from build123d import *

# Parameters (mm, degrees)
F0_W     = 50.8
F0_H     = 50.8
F1_DEPTH = 6.35
F2_W     = 50.8
F2_H     = 8.870684
F3_DEPTH = 6.604
F4_W     = 50.8
F4_H     = 50.8
F5_DEPTH = 6.35
F6_R     = 10.16
F6_R_2   = 8.255
F7_DEPTH = 50.8


with BuildPart() as f1:
    # F0 (on Top) → F1 (new body)
    with BuildSketch(Plane.XY):
        Rectangle(F0_W, F0_H)
    extrude(amount=F1_DEPTH)

    # F2 (on face) → F3 (join)
    with BuildSketch(Plane.XY.offset(6.35)):
        with Locations((0, 20.964658)):
            Rectangle(F2_W, F2_H)
    extrude(amount=F3_DEPTH)

    # F4 (on face) → F5 (join)
    with BuildSketch(Plane.XY.offset(12.954)):
        Rectangle(F4_W, F4_H)
    extrude(amount=F5_DEPTH)

    # F6 (on face) → F7 (join)
    with BuildSketch(Plane.XY.offset(19.304)):
        Circle(F6_R)
        Circle(F6_R_2, mode=Mode.SUBTRACT)
    extrude(amount=F7_DEPTH)


solid = f1.part
Geometry check sheet. Reference: the model listing, model coordinates, mm. A direction names the side the tool comes from. Round coordinates to 2 decimals unless told otherwise and drop trailing zeros. Order: outer loops, then holes, each group sorted by start corner. A loop starts at its lowest first (then second) coordinate and runs counter-clockwise, first axis right, second up. Notation, with made-up numbers: M 37,-33.75 L 51,-33.75 A21 cw 51,-23.75 Z; hole C 36,-30 d10. An arc over 180 degrees is marked long. Write each question's results on one line, items separated by ' | '. Start each with the question number.
1. Set-up check for faces 5 (the face through (0, -25.4, 3)), 6 (the face through (11, 0, 19.304)), 7 (the face through (0, -4, 6.35)): record each of +Z, -Z, +X, -X, +Y, -Y from which the full face is reachable in a straight line by a thin tool's end or side.
2. Cross-section at A-A on y = -19. Record the boundary of the cut face in (x, z), plus the area to 3 significant figures.
3. Cross-section at C-C on z = 32.5. Record the boundary of the cut face in (x, y) (3 decimals), plus the area to 3 significant figures.
4. Cross-section at B-B on x = 0. Record the boundary of the cut face in (y, z) (3 decimals), plus the area to 3 significant figures.
5. Go/stop test with flat-tipped pins: P1, Ø12, axis at y = 7.5, z = 58.5, coming from the +X side; P2, Ø3, axis at y = -10, z = 37.5, coming from the +X side; P3, Ø6, axis at x = -4.5, y = 18.5, coming from the +Z side. Record where each tip stops, or that it passes through.
6. Material ranges on L1, parallel to Y at x = 0, z = 49 (3 decimals); L2, parallel to Z at x = -5, y = 2; L3, parallel to X at y = -7, z = 42.5, recorded low to high. Write a range as from..to.
7. Cross-section at D-D on y = 0. Record the boundary of the cut face in (x, z) (3 decimals), plus the area to 3 significant figures.
8. Draft check along X on faces 1 (the face through (7.874, 2.48, 44.348)), 2 (the face through (0, 0, 19.304)), 3 (the face through (0, -25.4, 16)), 4 (the face through (25.4, 0, 14)). Enter one of: pulls with the +X half, pulls with the -X half, needs draft (parallel to the pull), parting line crosses it, or undercut.
Resolved:
1) face 5: +Z, -Z, +X, -X, -Y | face 6: +Z | face 7: +X, -X, -Y
2) outline: M -25.4,0 L 25.4,0 L 25.4,6.35 L -25.4,6.35 Z; M -25.4,12.95 L 25.4,12.95 L 25.4,19.3 L -25.4,19.3 Z | area: 645 mm2
3) outline: C 0,0 d20.32; hole C 0,0 d16.51 | area: 110 mm2
4) outline: M -25.4,0 L 25.4,0 L 25.4,19.304 L 10.16,19.304 L 10.16,70.104 L 8.255,70.104 L 8.255,19.304 L -8.255,19.304 L -8.255,70.104 L -10.16,70.104 L -10.16,19.304 L -25.4,19.304 L -25.4,12.954 L 16.529,12.954 L 16.529,6.35 L -25.4,6.35 Z | area: 897 mm2
5) P1: x = 10.05 | P2: x = 5.57 | P3: z = 19.3
6) L1: -10.16..-8.255, 8.255..10.16 | L2: 0..6.35, 12.95..19.3 | L3: -7.36..-4.38, 4.38..7.36
7) outline: M -25.4,0 L 25.4,0 L 25.4,6.35 L -25.4,6.35 Z; M -25.4,12.954 L 25.4,12.954 L 25.4,19.304 L 10.16,19.304 L 10.16,70.104 L 8.255,70.104 L 8.255,19.304 L -8.255,19.304 L -8.255,70.104 L -10.16,70.104 L -10.16,19.304 L -25.4,19.304 Z | area: 839 mm2
8) face 1: undercut | face 2: undercut | face 3: needs draft | face 4: pulls with the +X half
